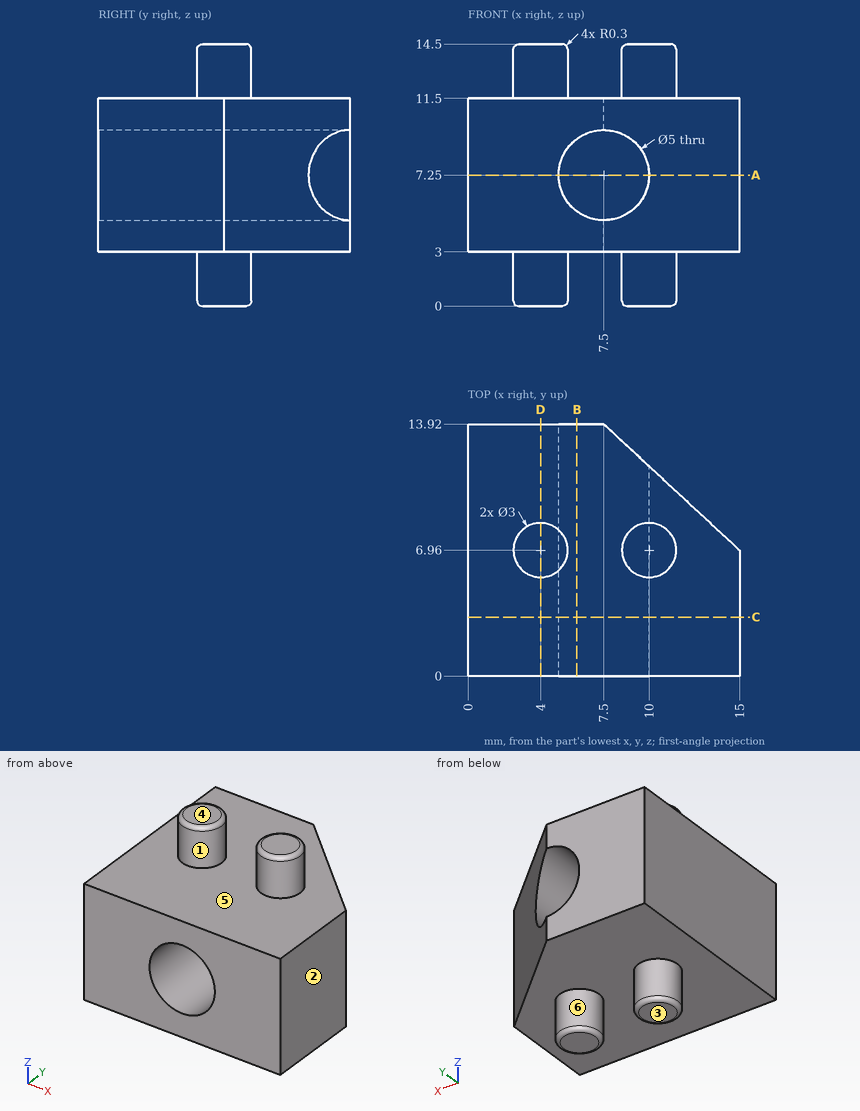
Here's the drawing with two shaded views (mm, measured from the low corner). I have some questions. A direction names the side the tool comes from. Give positions to 0.01 mm unless a question says otherwise; leave off trailing zeros. Loops run counter-clockwise (first coordinate to the right, second up) from the corner with the lowest first, then second, coordinate; pieces in that order, holes last. Notation, with made-up numbers: (48, 54) -> (54, 54) arc R25 ccw to (54, 74) -> close; hole circle Ø6 at (-37.75, -37). An arc over 180 degrees is marked (long way). One line per item, written item: value.
Q1. Suppose I cut it at D-D on x = 4. Please give me the cut outline in (y, z).
Answers follow:
outline: (0, 3) -> (5.46, 3) -> (5.46, 0.3) arc R0.3 ccw to (5.76, 0) -> (8.16, 0) arc R0.3 ccw to (8.46, 0.3) -> (8.46, 3) -> (13.92, 3) -> (13.92, 11.5) -> (8.46, 11.5) -> (8.46, 14.2) arc R0.3 ccw to (8.16, 14.5) -> (5.76, 14.5) arc R0.3 ccw to (5.46, 14.2) -> (5.46, 11.5) -> (0, 11.5) -> close
Q2. Suppose I cut it at A-A on z = 7.25. Please give me the cut outline in (x, y).
Answers follow:
outline: (0, 0) -> (5, 0) -> (5, 13.92) -> (0, 13.92) -> close; (10, 0) -> (15, 0) -> (15, 6.96) -> (10, 11.6) -> close
Q3. On a 3-axis mill with a long thin cutter (end or side, diameter ignored), from which of +Z, -Z, +X, -X, +Y, -Y can I reach the whole of each face in a straight line? I mean the marked faces 4, 5 and 6. Say none if no direction works.
Answers follow:
face 4: +Z, +X, -X, +Y, -Y
face 5: +Z
face 6: -Z
Q4. Suppose I cut it at B-B on x = 6. Please give me the cut outline in (y, z), then the cut area to 3 significant figures.
Answers follow:
outline: (0, 3) -> (13.92, 3) -> (13.92, 5.25) -> (0, 5.25) -> close; (0, 9.25) -> (13.92, 9.25) -> (13.92, 11.5) -> (0, 11.5) -> close
area: 62.6 mm^2
Q5. Suppose I cut it at C-C on y = 3.25. Please give me the cut outline in (x, z), then the cut area to 3 significant figures.
Answers follow:
outline: (0, 3) -> (15, 3) -> (15, 11.5) -> (0, 11.5) -> close; hole circle Ø5 at (7.5, 7.25)
area: 108 mm^2
Q6. I'm going to push flat-ended pins straight in: pin 1 Ø1.5 at (y, z) = (11.5, 8.5) entering from -X; pin 2 Ø1 at (x, y) = (13, 6.5) entering from -Z; pin 3 Ø2 at (x, z) = (9.5, 2.5) entering from +Y; pin 4 Ø6 at (x, y) = (9.5, 2) entering from +Z. Where does each tip first touch, or does it pass through?
Answers follow:
pin 1: x = 0
pin 2: z = 3
pin 3: y = 12.87
pin 4: z = 11.5
Q7. If I drill on line 1 along Z through (x, y) = (7.5, 6.5); line 2 along Z through (x, y) = (1.25, 3.25); line 3 along X through (y, z) = (5, 7.25), over which ranges is the centre line in solid material (lowest first)?
Answers follow:
line 1: 3 to 4.75, 9.75 to 11.5
line 2: 3 to 11.5
line 3: 0 to 5, 10 to 15
Q8. We'd pull the mould along X, two halves only. Please class the marked faces 1, 2 and 3: pulls with the +X half, pulls with the -X half, needs draft (parallel to the pull), parting line crosses it, or undercut.
Answers follow:
face 1: undercut
face 2: pulls with the +X half
face 3: needs draft
